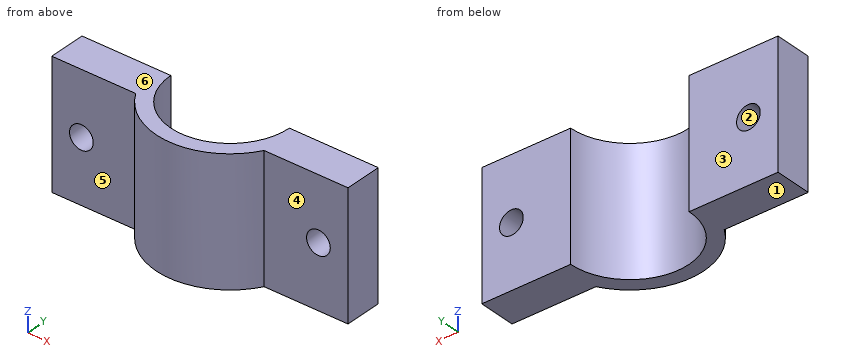
```python
from build123d import *

# Parameters (mm, degrees)
F1_DEPTH = 17
F2_R     = 1.6
F3_DEPTH = 25
F5_DEPTH = 25


with BuildPart() as f1:
    # F0 (on Top) → F1 (new body)
    with BuildSketch(Plane.XY):
        with BuildLine():
            Line((-8, 5), (-20, 5))
            Line((-20, 5), (-20, -5))
            Line((-20, -5), (20, -5))
            Line((20, -5), (20, 5))
            Line((20, 5), (8, 5))
            ThreePointArc((8, 5), (0, -3), (-8, 5))
        make_face()
    extrude(amount=F1_DEPTH)

    # F2 (on face) → F3 (cut)
    with BuildSketch(Plane.XZ.offset(5)):
        with Locations((-16, 8.5)):
            Circle(F2_R)
        with Locations((16, 8.5)):
            Circle(F2_R)
    extrude(amount=-F3_DEPTH, mode=Mode.SUBTRACT)

    # F4 (on face) → F5 (cut)
    with BuildSketch(Plane.XY.offset(17)):
        with BuildLine():
            ThreePointArc((8.660254, 0), (0, -5), (-8.660254, 0))
            Line((-8.660254, 0), (-20, 0))
            Line((-20, 0), (-20, -5.929414))
            Line((-20, -5.929414), (20, -5.929414))
            Line((20, -5.929414), (20, 0))
            Line((20, 0), (8.660254, 0))
        make_face()
    extrude(amount=-F5_DEPTH, mode=Mode.SUBTRACT)


solid = f1.part
```
Input: part model. Units: mm. Frame: model coordinates. Face numbers are marked on the shaded views. A direction names the side the tool comes from. Coordinates: 2 decimals unless noted, no trailing zeros. Order: outer loops, then holes, each group sorted by start corner. A loop starts at its lowest first (then second) coordinate and runs counter-clockwise, first axis right, second up. Notation, with made-up numbers: (-25.5, -5.75) - (6.5, -5.75) arc R21 cw to (6.5, 23.25) - close; hole circle Ø1 at (72, 17). An arc over 180 degrees is marked (long way). Return JSON: item names as keys, results as strings.
Q1. Cut plane B-B (z = 8.5). Return loops of the section in (x, y), then the cut area to 3 significant figures.
The answers:
{"outline": "(-20, 0) - (-17.6, 0) - (-17.6, 5) - (-20, 5) - close; (-14.4, 0) - (-8.66, 0) arc R10 ccw to (8.66, 0) - (14.4, 0) - (14.4, 5) - (8, 5) arc R8 cw to (-8, 5) - (-14.4, 5) - close; (17.6, 0) - (20, 0) - (20, 5) - (17.6, 5) - close", "area": "129 mm2"}
Q2. Access query for the marked faces 4, 5 and 6. Directions: +Z, -Z, +X, -X, +Y, -Y. A direction counts if a zero-diameter tool reaches every point of the face in a straight line with its end or side. Return the directions, or none.
The answers:
{"face 4": "+Z, -Z, +X, -Y", "face 5": "+Z, -Z, -X, -Y", "face 6": "+Z, +X, -X, +Y, -Y"}
Q3. Ray query, probe 1 along Z at (x, y) = (16, 2.25); probe 2 along Y at (x, z) = (-16.5, 13.25); probe 3 along Y at (x, z) = (0, 2.75). Return the intervals inside material, ascending.
The answers:
{"probe 1": "z = 0 to 6.9, 10.1 to 17", "probe 2": "y = 0 to 5", "probe 3": "y = -5 to -3"}
Q4. Cut plane A-A (y = 2). Return loops of the section in (x, z).
The answers:
{"outline": "(-20, 0) - (-7.42, 0) - (-7.42, 17) - (-20, 17) - close; (7.42, 0) - (20, 0) - (20, 17) - (7.42, 17) - close; hole circle Ø3.2 at (-16, 8.5); hole circle Ø3.2 at (16, 8.5)"}
Q5. First-contact query: pin 1 (8 mm diameter, centred on x = -9.5, z = 10, fed in from -Y); pin 2 (3.5 mm diameter, centred on x = -17, z = 7, fed in from -Y); pin 3 (1.5 mm diameter, centred on y = -2.5, z = 2, fed in from -X). Flat tips, straight axial feed; report the tip coordinate or a pass-through.
The answers:
{"pin 1": "stops at y = -3.35", "pin 2": "stops at y = 0", "pin 3": "stops at x = -7.38"}
Q6. Cut plane C-C (x = 16). Return loops of the section in (y, z), then the cut area to 3 significant figures.
The answers:
{"outline": "(0, 0) - (5, 0) - (5, 6.9) - (0, 6.9) - close; (0, 10.1) - (5, 10.1) - (5, 17) - (0, 17) - close", "area": "69.0 mm2"}
Q7. Draft query along Z for the marked faces 1, 2 and 3. Return one class per face: +Z half, -Z half, draft (parallel to the pull), parting line (faces both ways), or undercut.
The answers:
{"face 1": "-Z half", "face 2": "undercut", "face 3": "draft"}
Q8. Cut plane D-D (y = -2.5). Return loops of the section in (x, z).
The answers:
{"outline": "(-6.61, 0) - (-2.78, 0) - (-2.78, 17) - (-6.61, 17) - close; (2.78, 0) - (6.61, 0) - (6.61, 17) - (2.78, 17) - close"}
